```python
from build123d import *

# Parameters (mm, degrees)
F1_DEPTH = 50.8
F2_R     = 3.175
F4_W     = 6.35
F4_H     = 25.4
F5_DEPTH = 25.4


# Not quite as in the source:
# - two fillets or chamfers of one size are made in one step
# - a feature names something its author has since deleted; it is built from what else it names


with BuildPart() as f1:
    # F0 (on Front) → F1 (new body)
    with BuildSketch(Plane.XZ):
        Polygon((89.9496172311, 43.3501401251), (-160.8753827689, 43.3501401251), (-160.8753827689, 81.4501401251), (-113.2503827689, 81.4501401251), (-113.2503827689, 84.6251401251), (-164.0503827689, 84.6251401251), (-164.0503827689, 40.1751401251), (-113.2503827689, 40.1751401251), (39.1496172311, -102.6998598749), (89.9496172311, -102.6998598749), align=None)
        Polygon((-108.6081703534, 40.1751401251), (86.7746172311, 40.1751401251), (86.7746172311, -99.5248598749), (40.4051629799, -99.5248598749), align=None, mode=Mode.SUBTRACT)
    extrude(amount=F1_DEPTH)

    # F2
    f2_edges = [f1.edges().sort_by_distance(p)[0] for p in [
        (-164.050383, -25.4, 84.62514),
        (-160.875383, -25.4, 43.35014),
        (89.949617, -25.4, 43.35014),
        (89.949617, -25.4, -102.69986),
        (-164.050383, -25.4, 40.17514),
        (-160.875383, -25.4, 81.45014),
        (39.149617, -25.4, -102.69986),
        (40.405163, -25.4, -99.52486),
        (86.774617, -25.4, 40.17514),
        (86.774617, -25.4, -99.52486),
    ]]
    fillet(f2_edges, radius=F2_R)

    # F4 (on face) → F5 (cut)
    with BuildSketch(Plane.YZ.offset(89.9496172311)):
        with Locations((-3.175, 21.1251401251)):
            Rectangle(F4_W, F4_H)
        with Locations((-47.625, 21.1251401251)):
            Rectangle(F4_W, F4_H)
    extrude(amount=-F5_DEPTH, mode=Mode.SUBTRACT)


solid = f1.part
```
For this review, take the finished solid that the model builds, in its own axes (mm). A direction names the side the tool comes from. Round coordinates to 2 decimals unless told otherwise and drop trailing zeros. Write each loop counter-clockwise with the first axis right and the second up, starting at its lowest first coordinate (ties: lowest second). Pieces come first, ordered by that corner, then holes. Notation, with made-up numbers: M -30,89.5 L 13,89.5 A17 cw 13,100.5 Z; hole C 69,-0.75 d7. An arc over 180 degrees is marked long. One line per item, written item: value. Start each with the question number.
(1) We need section C-C (z = -16). Give the boundary of the cut face in (x, y), and give its area (3 significant figures).
(2) Insertion check: pin 1 (2.5 mm diameter, centred on x = 88.5, y = -47.5, fed in from +Z); pin 2 (13.5 mm diameter, centred on x = -139.5, y = -24, fed in from -Z); pin 3 (6 mm diameter, centred on x = -81, y = -14, fed in from +Z). Each pin has a flat end and moves straight along its axis. Give the tip position at first contact, or say it passes through.
(3) Wall thickness on line 1 (Z direction, x = -143.5, y = -43); line 2 (X direction, y = -47, z = 61); line 3 (X direction, y = -39, z = -51.5): over which ranges is each line inside the solid? List them lowest first.
(4) We need section B-B (y = -33.5). Give the boundary of the cut face in (x, z) (3 decimals).
(5) Machinability: for faces 1 (the flat face through (-137, -25, 40.175)), 2 (the flat face through (-137, -25, 84.625)), 3 (the flat face through (86.775, -25, -29)), 4 (the flat face through (-136, -25, 81.45)), which of the approach directions +Z, -Z, +X, -X, +Y, -Y give a long, thin tool a straight path to every point of the face, cutting with its end or side? Answer none if there is none.
(6) We need section A-A (x = -138.5). Give the boundary of the cut face in (y, z).
(7) The part is to be moulded in two halves that separate along X. For faces 5 (the flat face through (-75, -50.8, 5)), 6 (the flat face through (-33.52, -25.04, -30.22)), 7 (the flat face through (-38.57, -25.04, -29.84)), say which applies: released by +X, released by -X, zero draft, split by the parting line, or undercut.
Result:
1. outline: M -53.33,-50.8 L -48.69,-50.8 L -48.69,0 L -53.33,0 Z; M 86.77,-50.8 L 89.95,-50.8 L 89.95,0 L 86.77,0 Z
1. area: 397 mm²
2. pin 1: z = 43.31
2. pin 2: z = 40.18
2. pin 3: z = 43.35
3. line 1: 40.18 to 43.35, 81.45 to 84.63
3. line 2: -164.05 to -160.88
3. line 3: -15.46 to -10.82, 86.77 to 89.95
4. outline: M -164.05,43.35 A3.175 ccw -160.875,40.175 L -113.25,40.175 L 38.234,-101.841 A3.175 ccw 40.405,-102.7 L 86.775,-102.7 A3.175 ccw 89.95,-99.525 L 89.95,40.175 A3.175 ccw 86.775,43.35 L -157.7,43.35 A3.175 cw -160.875,46.525 L -160.875,78.275 A3.175 cw -157.7,81.45 L -113.25,81.45 L -113.25,84.625 L -160.875,84.625 A3.175 ccw -164.05,81.45 Z; hole M -108.608,40.175 L 39.489,-98.666 A3.175 ccw 41.661,-99.525 L 83.6,-99.525 A3.175 ccw 86.775,-96.35 L 86.775,37 A3.175 ccw 83.6,40.175 Z
5. face 1: -Z, -X, +Y, -Y
5. face 2: +Z, +X, -X, +Y, -Y
5. face 3: +Y, -Y
5. face 4: +X, +Y, -Y
6. outline: M -50.8,40.18 L 0,40.18 L 0,43.35 L -50.8,43.35 Z; M -50.8,81.45 L 0,81.45 L 0,84.63 L -50.8,84.63 Z
7. face 5: zero draft
7. face 6: undercut
7. face 7: released by -X
